Autodesk Inventor part; units mm, degrees
ref_plane "YZ Plane" through (0, 0, 0) normal (1, 0, 0) x (0, 1, 0)
ref_plane "XZ Plane" through (0, 0, 0) normal (0, 1, 0) x (-1, 0, 0)
ref_plane "XY Plane" through (0, 0, 0) normal (0, 0, 1) x (1, 0, 0)
sketch "Sketch1" plane through (0, 0, 0) normal (0, 1, 0) x (-1, 0, 0)
  line L0 (51.1762, 45) -> (-51.1762, 45)
  line L1 (12, -62.25) -> (-12, -62.25)
  line L2 (-12, -60) -> (12, -60)
  circle A0 centre (0, 0) radius 6
  circle A1 centre (-44.3523, -52.8571) radius 1.5 construction
  circle A2 centre (-41.7906, 34.5) radius 1.5
  circle A3 centre (-62.5352, -29.1607) radius 1.5
  circle A4 centre (62.5352, -29.1607) radius 1.5
  circle A5 centre (-20, 41.5) radius 1.5 construction
  circle A6 centre (41.7906, 34.5) radius 1.5
  circle A7 centre (20, 41.5) radius 1.5 construction
  circle A8 centre (44.3523, -52.8571) radius 1.5 construction
  arc A9 (12, -62.25) -> (12, -60) centre (12, -61.125) ccw
  arc A10 (-12, -60) -> (-12, -62.25) centre (-12, -61.125) ccw
  circle A11 centre (0, 0) radius 69 construction
  line L3 (0, 0) -> (0, 45)
  arc A12 (-59.4304, 40.6452) -> (59.4304, 40.6452) centre (0, 0) ccw
  arc A13 (-51.1762, 45) -> (-59.4304, 40.6452) centre (-51.1762, 35) ccw
  arc A14 (59.4304, 40.6452) -> (51.1762, 45) centre (51.1762, 35) ccw
  line L4 (0, 0) -> (-72, 0)
  line L5 (0, 0) -> (62.5352, -29.1607) construction
  line L6 (0, 0) -> (69, 0)
  line L7 (0, 0) -> (41.7906, 34.5) construction
  line L8 (47.057, 23.5) -> (68.057, 23.5)
  line L9 (68.057, 23.5) -> (68.057, -23.5)
  line L10 (68.057, -23.5) -> (47.057, -23.5)
  line L11 (47.057, -23.5) -> (47.057, 23.5)
  line L12 (47.057, 23.5) -> (68.057, -23.5) construction
  line L13 (68.057, 23.5) -> (47.057, -23.5) construction
  circle A15 centre (38.657, -9) radius 1
  circle A16 centre (38.657, 9) radius 1
  circle A17 centre (16, -12.35) radius 1.5
  circle A18 centre (33.75, -59) radius 1.5
  circle A19 centre (-16, -12.35) radius 1.5
  circle A20 centre (-33.75, -59) radius 1.5
  line L14 (-47.057, 23.5) -> (-68.057, 23.5)
  line L15 (-68.057, 23.5) -> (-68.057, -23.5)
  line L16 (-68.057, -23.5) -> (-47.057, -23.5)
  line L17 (-47.057, -23.5) -> (-47.057, 23.5)
  circle A21 centre (-38.657, -9) radius 1
  circle A22 centre (-38.657, 9) radius 1
  line L18 (39, -25.5) -> (33, -25.5)
  line L19 (33, -25.5) -> (33, -36.5)
  line L20 (33, -36.5) -> (39, -36.5)
  line L21 (39, -36.5) -> (39, -25.5)
  circle A23 centre (36, -38.5) radius 1
  line L22 (39, -31) -> (33, -31)
  circle A24 centre (36, -23.5) radius 1
  circle A25 centre (40.817, -45.3318) radius 1.5
  circle A26 centre (-41.7906, 34.5) radius 1.5
  circle A27 centre (-40.817, -45.3318) radius 1.5
  line L23 (41.7906, 34.5) -> (41.7906, 39.5)
  line L24 (41.7906, 39.5) -> (60.1976, 39.5) construction
  line L25 (0, 0) -> (44.3523, -52.8571) construction
  circle A28 centre (62.5352, 29.1607) radius 1.5
  circle A29 centre (-62.5352, 29.1607) radius 1.5
  line L26 (40.817, -45.3318) -> (0, 0) construction
  line L27 (0, 0) -> (62.5352, 29.1607) construction
  circle A30 centre (10, 6) radius 1.5
  circle A31 centre (-10, 6) radius 1.5
  line L28 (33.2906, 29.5) -> (34.2906, 29.5)
  line L29 (36.2906, 27.5) -> (36.2906, 21.5)
  line L30 (34.2906, 19.5) -> (33.2906, 19.5)
  line L31 (31.2906, 21.5) -> (31.2906, 27.5)
  arc A32 (34.2906, 19.5) -> (36.2906, 21.5) centre (34.2906, 21.5) ccw
  arc A33 (31.2906, 21.5) -> (33.2906, 19.5) centre (33.2906, 21.5) ccw
  arc A34 (33.2906, 29.5) -> (31.2906, 27.5) centre (33.2906, 27.5) ccw
  arc A35 (36.2906, 27.5) -> (34.2906, 29.5) centre (34.2906, 27.5) ccw
  line L32 (0, 0) -> (-41.7906, 34.5) construction
  line L33 (-33.2906, 29.5) -> (-34.2906, 29.5)
  line L34 (-36.2906, 27.5) -> (-36.2906, 21.5)
  line L35 (-34.2906, 19.5) -> (-33.2906, 19.5)
  line L36 (-31.2906, 21.5) -> (-31.2906, 27.5)
  arc A36 (-36.2906, 21.5) -> (-34.2906, 19.5) centre (-34.2906, 21.5) ccw
  arc A37 (-33.2906, 19.5) -> (-31.2906, 21.5) centre (-33.2906, 21.5) ccw
  arc A38 (-31.2906, 27.5) -> (-33.2906, 29.5) centre (-33.2906, 27.5) ccw
  arc A39 (-34.2906, 29.5) -> (-36.2906, 27.5) centre (-34.2906, 27.5) ccw
  circle A40 centre (0, 0) radius 54.1913
  circle A41 centre (0, 0) radius 61 construction
  point P0 (-5.9883, -61.0615)
  point P1 (57.557, 0)
  point P2 (68.057, 23.5)
  point P3 (-68.057, 23.5)
  point P4 (-68.057, -23.5)
  point P5 (0, 34.5)
  point P6 (36, -36.5)
  point P7 (55.8424, 43.8445)
  point P8 (0, -6)
  point P9 (31.2906, 29.5)
  point P10 (31.2906, 19.5)
  point P11 (33.7906, 29.5)
  point P12 (-31.2906, 29.5)
  point P13 (-31.2906, 19.5)
  point P14 (-33.7906, 29.5)
  dimension "d12" = 12
  dimension "d398" = 108.3827
  dimension "d0" = 3
  dimension "d1" = 3
  dimension "d4" = 3
  dimension "d15" = 24
  dimension "d16" = 3
  dimension "d62" = 2.25
  dimension "d148" = 3.5
  dimension "d276" = 138
  dimension "d285" = 144
  dimension "d286" = 45
  dimension "d287" = 10
  dimension "d288" = 12
  dimension "d289" = 40
  dimension "d290" = 3.5
  dimension "d291" = 20
  dimension "d293" = 25
  dimension "d300" = 21
  dimension "d301" = 47
  dimension "d304" = 2
  dimension "d305" = 8.4
  dimension "d306" = 9
  dimension "d307" = 3
  dimension "d311" = 16
  dimension "d318" = 33.75
  dimension "d323" = 11
  dimension "d324" = 6
  dimension "d325" = 2
  dimension "d326" = 2
  dimension "d327" = 15
  dimension "d338" = 33
  dimension "d342" = 5
  dimension "d345" = 11
  dimension "d346" = 39.541
  dimension "d348" = 40
  dimension "d350" = 61
  dimension "d351" = 48
  dimension "d352" = 3
  dimension "d353" = 12.35
  dimension "d354" = 59
  dimension "d355" = 25
  dimension "d356" = 60
  dimension "d358" = 68.057
  dimension "d371" = 3
  dimension "d372" = 10
  dimension "d373" = 6
  dimension "d393" = 5
  dimension "d394" = 10
  dimension "d395" = 5
  dimension "d396" = 2
  dimension "d397" = 8
extrude "Extrusion1" add sketch "Sketch1" along normal blind 3 contours A14 A12 L8 A40 A6 L0 | A40 A6 L8 L11 L6 A0 L3 L0 | L3 A0 L4 L17 L14 A40 A2 L0 | A40 A2 L14 A12 A13 L0 | A12 L16 A40 L10 | L6 L11 L10 A40 L16 L17 L4 A0
sketch "Sketch3" plane through (0, 3, 0) normal (0, 1, 0) x (1, 0, 0)
  line L0 (3, 0) -> (3, -20)
  circle A0 centre (-10.775, -23.1) radius 1.5
  line L1 (-51.1762, -45) -> (51.1762, -45)
  circle A1 centre (16.775, -30.6) radius 1.5
  point P0 (0, 0)
  dimension "d377" = 20
  dimension "d378" = 3
  dimension "d379" = 3
  dimension "d380" = 13.775
  dimension "d381" = 21.9
  dimension "d383" = 13.775
  dimension "d384" = 3
  dimension "d385" = 14.4
fillet "Fillet1" radius 2 1 edges at (68.057, 1.5, 23.5)
fillet "Fillet2" radius 2 7 edges at (68.057, 1.5, -23.5) (-68.057, 1.5, -23.5) (-68.057, 1.5, 23.5) (-47.057, 1.5, -23.5) (-47.057, 1.5, 23.5) (47.057, 1.5, -23.5) (47.057, 1.5, 23.5)
sketch "Sketch2" plane through (0, 3, 0) normal (0, 1, 0) x (1, 0, 0)
  circle A0 centre (62.5352, 29.1607) radius 1.5
  circle A1 centre (62.5352, -29.1607) radius 1.5
  line L0 (62.5352, 29.1607) -> (62.5352, -29.1607)
  line L1 (62.5352, -29.1607) -> (62.5352, -30.3154)
  line L2 (62.5352, -27.1607) -> (61.0352, -27.1607)
  line L3 (-51.1762, -45) -> (51.1762, -45)
  line L4 (0, -45) -> (0, 72)
  arc A2 (67.0527, 26.2286) -> (-67.0527, 26.2286) centre (0, 0) ccw
  line L5 (59.4352, -31.1607) -> (59.4352, -27.1607)
  line L6 (59.4352, -27.1607) -> (61.0352, -27.1607)
  line L7 (62.5352, -27.1607) -> (62.5352, -30.3154)
  line L8 (59.4352, -31.1607) -> (59.4352, -32.6607)
  line L9 (59.4352, -32.6607) -> (62.5352, -32.6607)
  line L10 (62.5352, -32.6607) -> (62.5352, -30.3154)
  line L11 (62.5352, -29.1607) -> (59.4352, -29.1607)
  line L12 (-70, 0) -> (70, 0)
  line L13 (62.5352, 29.1607) -> (62.5352, 30.3154)
  line L14 (62.5352, 27.1607) -> (61.0352, 27.1607)
  line L15 (59.4352, 31.1607) -> (59.4352, 27.1607)
  line L16 (59.4352, 27.1607) -> (61.0352, 27.1607)
  line L17 (62.5352, 27.1607) -> (62.5352, 30.3154)
  line L18 (59.4352, 31.1607) -> (59.4352, 32.6607)
  line L19 (59.4352, 32.6607) -> (62.5352, 32.6607)
  line L20 (62.5352, 32.6607) -> (62.5352, 30.3154)
  line L21 (-62.5352, -27.1607) -> (-61.0352, -27.1607)
  line L22 (-59.4352, -31.1607) -> (-59.4352, -27.1607)
  line L23 (-59.4352, -27.1607) -> (-61.0352, -27.1607)
  line L24 (-62.5352, -27.1607) -> (-62.5352, -30.3154)
  line L25 (-59.4352, -31.1607) -> (-59.4352, -32.6607)
  line L26 (-59.4352, -32.6607) -> (-62.5352, -32.6607)
  line L27 (-62.5352, -32.6607) -> (-62.5352, -30.3154)
  line L28 (-62.5352, -29.1607) -> (-59.4352, -29.1607)
  line L29 (-59.4352, 32.6607) -> (-62.5352, 32.6607)
  line L30 (-59.4352, 31.1607) -> (-59.4352, 32.6607)
  line L31 (-59.4352, 31.1607) -> (-59.4352, 27.1607)
  line L32 (-59.4352, 27.1607) -> (-61.0352, 27.1607)
  line L33 (-62.5352, 27.1607) -> (-61.0352, 27.1607)
  line L34 (-62.5352, 32.6607) -> (-62.5352, 30.3154)
  line L35 (-62.5352, 29.1607) -> (-62.5352, 30.3154)
  line L36 (-62.5352, 27.1607) -> (-62.5352, 30.3154)
  line L37 (-62.5352, 29.1607) -> (-59.4352, 29.1607)
  line L38 (62.5352, 29.1607) -> (59.4352, 29.1607)
  point P0 (62.5352, 27.1607)
  point P1 (62.5352, 27.6607)
  point P2 (60.7226, 29.8154)
  point P3 (60.7226, -29.8154)
  point P4 (62.5352, -27.6607)
  point P5 (62.5352, -27.1607)
  point P6 (62.5352, 30.6607)
  point P7 (62.5352, -30.6607)
  dimension "d363" = 1.5
  dimension "d365" = 4
  dimension "d366" = 1.5
  dimension "d367" = 3.1
  dimension "d368" = 1.6
extrude "Extrusion2" [suppressed]
hole "Hole1" at (-10.775, 3, 23.1) at (16.775, 3, 30.6) direction (0, -1, 0) diameter 3 end through all
properties part number "base_chasis_v6"
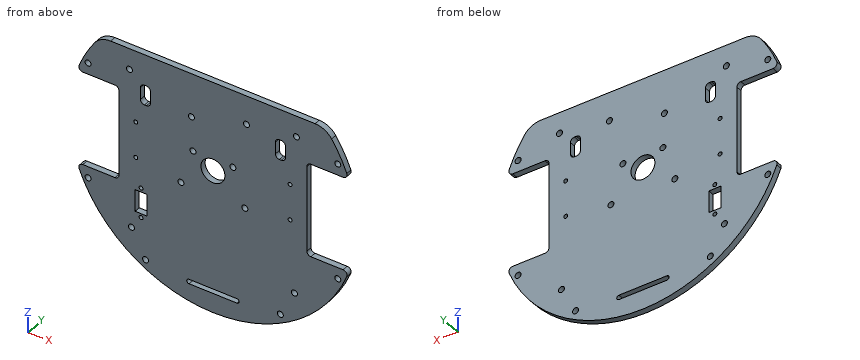
Could you check a few things on this model? Use its own coordinates, in mm. Round coordinates to 2 decimals unless told otherwise and drop trailing zeros. Order: outer loops, then holes, each group sorted by start corner. A loop starts at its lowest first (then second) coordinate and runs counter-clockwise, first axis right, second up. Notation, with made-up numbers: M 6.25,76 L 42.25,76 A7 cw 42.25,84 Z; hole C 76.5,17 d6. An arc over 180 degrees is marked long. One line per question, with ' | ' between items. Start each with the question number.
(1) Suppose I cut it at C-C on x = -16. List the corners of the cut face in (y, z) for me, then the cut area to 3 significant figures.
(2) Please list where these lines run through material, in increasing order: line 1 along X through (y, z) = (1.35, 34.5); line 2 along Z through (x, y) = (-9, 2.15); line 3 along Z through (x, y) = (-4.5, 0.9).
(3) Suppose I cut it at B-B on z = -12.35. List the corners of the cut face in (x, y) for me, then the cut area to 3 significant figures.
(4) Suppose I cut it at A-A on x = 0. List the corners of the cut face in (y, z) for me, then the cut area to 3 significant figures.
(5) Suppose I cut it at D-D on z = 12.5. List the corners of the cut face in (x, y) for me, then the cut area to 3 significant figures.
(6) For P1, Ø0.9, axis at x = 55, y = 2, coming from the -Z side; P2, Ø1.5, axis at y = 2, z = -32.5, coming from the -X side; P3, Ø1.5, axis at y = 1, z = -49, coming from the -X side, each with a flat end and sliding along its axis, tell me the tip position at first contact or that it passes through.
Geometry results:
1) outline: M 0,-70.2 L 3,-70.2 L 3,-13.85 L 0,-13.85 Z; M 0,-10.85 L 3,-10.85 L 3,45 L 0,45 Z | area: 337 mm²
2) line 1: -63.2 to -43.29, -40.29 to 40.29, 43.29 to 63.2 | line 2: -71.44 to -62.25, -60 to 4.88, 7.12 to 45 | line 3: -71.86 to -62.25, -60 to -3.97, 3.97 to 45
3) outline: M -47.06,0 L -17.5,0 L -17.5,3 L -47.06,3 Z; M -14.5,0 L 14.5,0 L 14.5,3 L -14.5,3 Z; M 17.5,0 L 47.06,0 L 47.06,3 L 17.5,3 Z | area: 264 mm²
4) outline: M 0,-72 L 3,-72 L 3,-62.25 L 0,-62.25 Z; M 0,-60 L 3,-60 L 3,-6 L 0,-6 Z; M 0,6 L 3,6 L 3,45 L 0,45 Z | area: 308 mm²
5) outline: M -47.06,0 L 47.06,0 L 47.06,3 L -47.06,3 Z | area: 282 mm²
6) P1: z = -46.99 | P2: x = -64.62 | P3: x = -53.44
